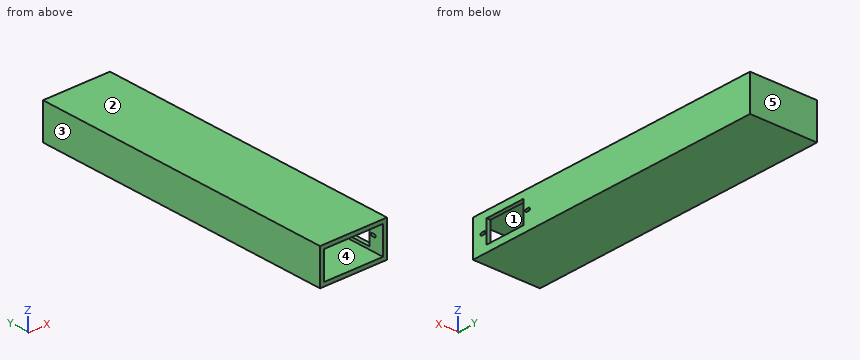
from build123d import *

# Parameters (mm, degrees)
SKETCH007_W     = 37.5
SKETCH007_H     = 172.3
PAD002_DEPTH    = 20
SKETCH006_W     = 33.1
SKETCH006_H     = 15.6
POCKET004_DEPTH = 172
SKETCH009_W     = 23
SKETCH009_H     = 12.5
POCKET003_DEPTH = 10
POCKET005_DEPTH = 5


with BuildPart() as part:
    # Sketch007 → Pad002 (new body)
    with BuildSketch(Plane.XY):
        Rectangle(SKETCH007_W, SKETCH007_H)
    extrude(amount=PAD002_DEPTH)

    # Sketch006 (on Face1 of Pad002) → Pocket004 (cut)
    with BuildSketch(Plane.XZ.offset(86.15)):
        with Locations((0, 10)):
            Rectangle(SKETCH006_W, SKETCH006_H)
    extrude(amount=-POCKET004_DEPTH, mode=Mode.SUBTRACT)

    # Sketch009 (on Face5 of Pocket004) → Pocket003 (cut)
    with BuildSketch(Plane.YZ.offset(18.75)):
        with Locations((-66.15, 10)):
            Rectangle(SKETCH009_W, SKETCH009_H)
    extrude(amount=-POCKET003_DEPTH, mode=Mode.SUBTRACT)

    # Sketch005 (on Face5 of Pocket003) → Pocket005 (cut)
    with BuildSketch(Plane.YZ.offset(18.75)):
        with BuildLine():
            ThreePointArc((-80.775673, 10.75), (-81.525673, 10), (-80.775673, 9.25))
            Line((-80.775673, 9.25), (-79.275673, 9.25))
            ThreePointArc((-79.275673, 9.25), (-78.525673, 10), (-79.275673, 10.75))
            Line((-80.775673, 10.75), (-79.275673, 10.75))
        make_face()
        with BuildLine():
            ThreePointArc((-52.955318, 10.75), (-53.705318, 10), (-52.955318, 9.25))
            Line((-52.955318, 9.25), (-51.455318, 9.25))
            ThreePointArc((-51.455318, 9.25), (-50.705318, 10), (-51.455318, 10.75))
            Line((-52.955318, 10.75), (-51.455318, 10.75))
        make_face()
    extrude(amount=-POCKET005_DEPTH, mode=Mode.SUBTRACT)


solid = part.part
Read the model definition and answer for the solid it produces. Units are mm, in the model's axes. Face numbers are marked on the shaded views. A direction names the side the tool comes from. Round coordinates to 2 decimals unless told otherwise and drop trailing zeros. Write each loop counter-clockwise with the first axis right and the second up, starting at its lowest first coordinate (ties: lowest second). Pieces come first, ordered by that corner, then holes. Notation, with made-up numbers: (55, 57) - (90, 57) arc R20 ccw to (90, 70) - close; hole circle Ø4 at (53.5, 7). An arc over 180 degrees is marked (long way). Use a Markdown table: item, result.
(1) The part is cut by section B-B (x = 9.5). Write down the section's boundary in (y, z).
Reported:
| item | result |
|---|---|
| outline | (-86.15, 0) - (86.15, 0) - (86.15, 20) - (-86.15, 20) - (-86.15, 17.8) - (85.85, 17.8) - (85.85, 2.2) - (-86.15, 2.2) - close |
(2) The part is cut by section A-A (y = 76). Write down the section's boundary in (x, z), then the cut area to 3 significant figures.
Reported:
| item | result |
|---|---|
| outline | (-18.75, 0) - (18.75, 0) - (18.75, 20) - (-18.75, 20) - close; hole (-16.55, 2.2) - (16.55, 2.2) - (16.55, 17.8) - (-16.55, 17.8) - close |
| area | 234 mm2 |
(3) Each of these flat-tipped pins is pushed along its axis until it touches: pin 1 Ø1 at (x, y) = (10.5, -52.5) entering from -Z; pin 2 Ø1.5 at (x, z) = (10.5, 17) entering from -Y. Where does it stop, or does it pass through?
Reported:
| item | result |
|---|---|
| pin 1 | z = 0 |
| pin 2 | y = 85.85 |
(4) The mould has two halves that part along X. Classify the marked faces 3, 4 and 5: released by +X, released by -X, zero draft, split by the parting line, or undercut.
Reported:
| item | result |
|---|---|
| face 3 | released by -X |
| face 4 | undercut |
| face 5 | zero draft |
(5) The part is cut by section C-C (y = -59). Write down the section's boundary in (x, z), then the cut area to 3 significant figures.
Reported:
| item | result |
|---|---|
| outline | (-18.75, 0) - (18.75, 0) - (18.75, 3.75) - (16.55, 3.75) - (16.55, 2.2) - (-16.55, 2.2) - (-16.55, 17.8) - (16.55, 17.8) - (16.55, 16.25) - (18.75, 16.25) - (18.75, 20) - (-18.75, 20) - close |
| area | 206 mm2 |
(6) Which of the six approach directions +Z, -Z, +X, -X, +Y, -Y give full straight-line access (tool end or side, diameter ignored) to the marked faces 1 and 2?
Reported:
| item | result |
|---|---|
| face 1 | -Y |
| face 2 | +Z, +X, -X, +Y, -Y |
(7) Straight lines are drawn through the part: line 1 along X through (y, z) = (-67, 16.5); line 2 along Z through (x, y) = (-2, 55); line 3 along Y through (x, z) = (9.5, 3.25). For each, find the intervals that lie inside material, in ascending order. Write a range as [from, to].
Reported:
| item | result |
|---|---|
| line 1 | [-18.75, -16.55], [16.55, 18.75] |
| line 2 | [0, 2.2], [17.8, 20] |
| line 3 | [85.85, 86.15] |
